Job drawing, mm, ordinate dimensions from the low corner. One solid piece. Give positions to 0.01 mm unless a question says otherwise; leave off trailing zeros. Write each loop counter-clockwise with the first axis right and the second up, starting at its lowest first coordinate (ties: lowest second). Pieces come first, ordered by that corner, then holes. Notation, with made-up numbers: M 31,56.25 L 79,56.25 A14 ccw 79,80.25 Z; hole C 5,-33 d11. An arc over 180 degrees is marked long. Answer as CSV lines item,"result". Start each with the question number.
1) Slice it at C-C, the plane y = 4.3. Give the cut face in (x, z).
2) Slice it at B-B, the plane z = 3.5. Give the cut face in (x, y).
3) Pin check, flat tips, straight feed: pin 1 Ø3.5 at (x, z) = (8, 3.5) entering from -Y; pin 2 Ø2.5 at (x, z) = (77, 3.5) entering from +Y. Stop position of each tip, or through.
4) Wall check: line 1 along X through (y, z) = (0.75, 3.5); line 2 along X through (y, z) = (4, 3.5); line 3 along Z through (x, y) = (8, 1.15). Give the ranges that are in metal, low to high. Write a range as from..to.
5) Slice it at A-A, the plane x = 77. Give the cut face in (y, z).
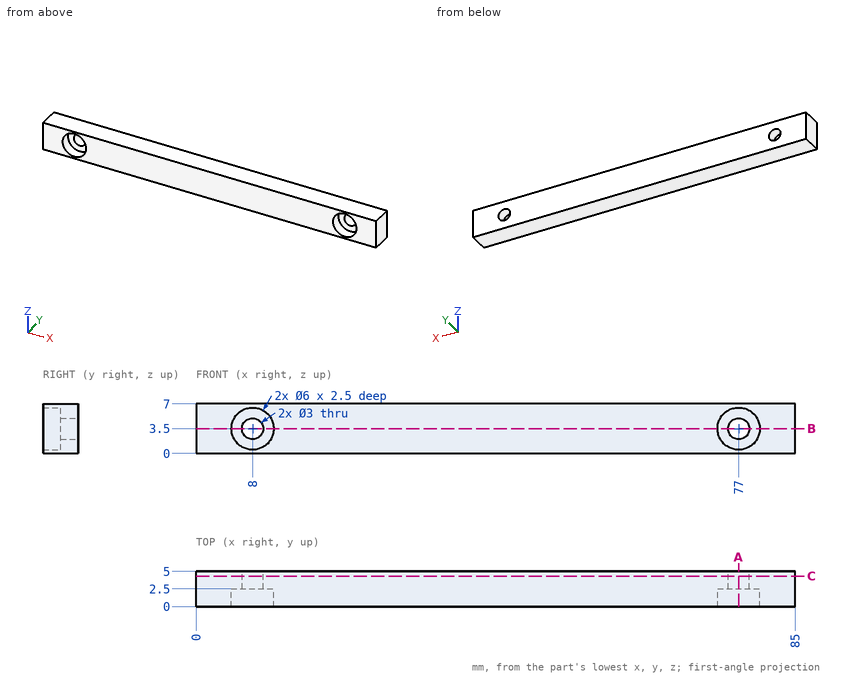
Found:
1,outline,"M 0,0 L 85,0 L 85,7 L 0,7 Z; hole C 8,3.5 d3; hole C 77,3.5 d3"
2,outline,"M 0,0 L 5,0 L 5,2.5 L 6.5,2.5 L 6.5,5 L 0,5 Z; M 9.5,2.5 L 11,2.5 L 11,0 L 74,0 L 74,2.5 L 75.5,2.5 L 75.5,5 L 9.5,5 Z; M 78.5,2.5 L 80,2.5 L 80,0 L 85,0 L 85,5 L 78.5,5 Z"
3,pin 1,"y = 2.5"
3,pin 2,"through"
4,line 1,"0..5, 11..74, 80..85"
4,line 2,"0..6.5, 9.5..75.5, 78.5..85"
4,line 3,"0..0.5, 6.5..7"
5,outline,"M 0,0 L 5,0 L 5,2 L 2.5,2 L 2.5,0.5 L 0,0.5 Z; M 0,6.5 L 2.5,6.5 L 2.5,5 L 5,5 L 5,7 L 0,7 Z"
